For this review, use the dimensioned drawing (mm, ordinates from the lowest corner) and the shaded views. Round coordinates to 2 decimals unless told otherwise and drop trailing zeros. Write each loop counter-clockwise with the first axis right and the second up, starting at its lowest first coordinate (ties: lowest second). Pieces come first, ordered by that corner, then holes. Notation, with made-up numbers: (88.25, 44) - (97.25, 44) arc R7 cw to (97.25, 51) - close; hole circle Ø1 at (53, 46). An arc over 180 degrees is marked (long way). Return JSON: item names as keys, results as strings.
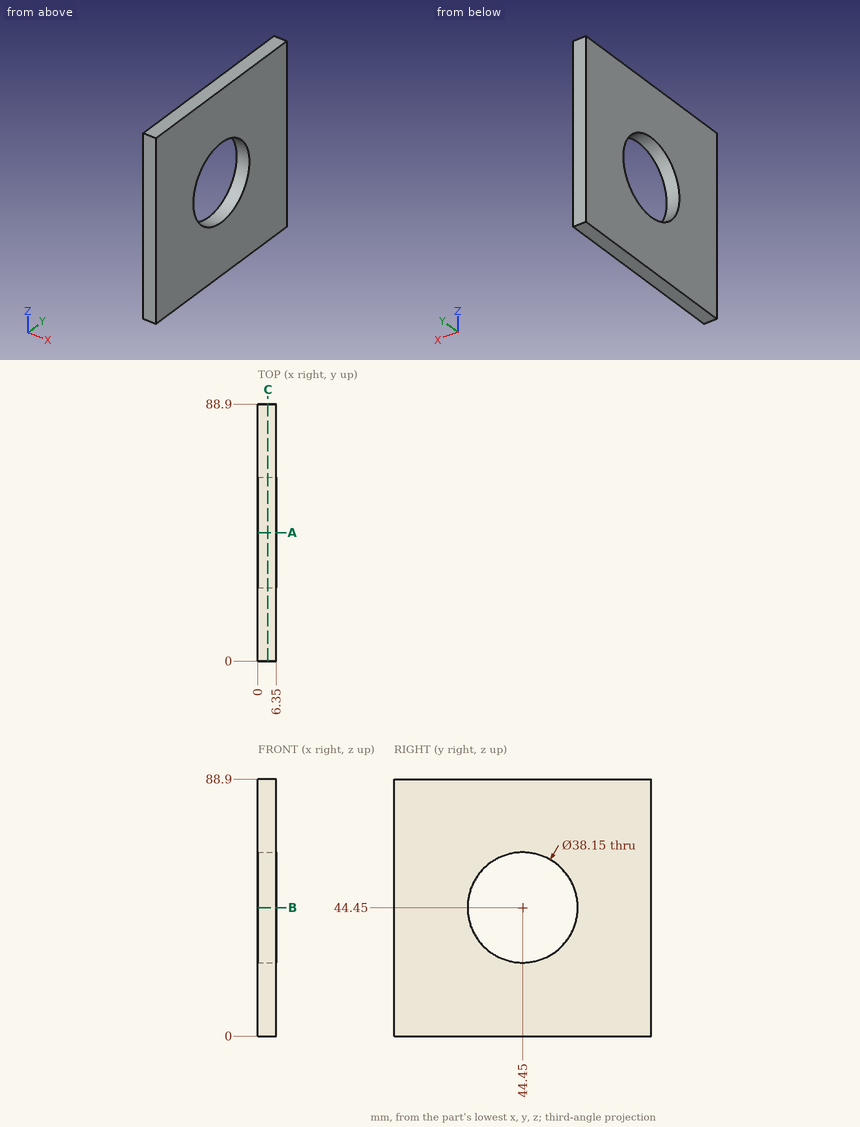
(1) Clearance check with flat-ended pins moving along their axes: pin 1 Ø2 at (x, z) = (2.5, 51) entering from -Y; pin 2 Ø3 at (y, z) = (43, 60) entering from -X. State where each tip first meets the part, or that it passes through.
Filled in:
{"pin 1": "stops at y = 0", "pin 2": "passes through"}
(2) Add section C-C (x = 3.5). Write out the cut boundary in (y, z) (3 decimals).
Filled in:
{"outline": "(0, 0) - (88.9, 0) - (88.9, 88.9) - (0, 88.9) - close; hole circle Ø38.15 at (44.45, 44.45)"}
(3) Wall thickness on line 1 (Z direction, x = 2, y = 44.45) (3 decimals); line 2 (Y direction, x = 2, z = 52); line 3 (Z direction, x = 6.25, y = 38): over which ranges is each line inside the solid? List them lowest first.
Filled in:
{"line 1": "z = 0 to 25.375, 63.525 to 88.9", "line 2": "y = 0 to 26.93, 61.97 to 88.9", "line 3": "z = 0 to 26.5, 62.4 to 88.9"}
(4) Add section A-A (y = 44.45). Write out the cut boundary in (x, z) (3 decimals), plus the area to 3 significant figures.
Filled in:
{"outline": "(0, 0) - (6.35, 0) - (6.35, 25.375) - (0, 25.375) - close; (0, 63.525) - (6.35, 63.525) - (6.35, 88.9) - (0, 88.9) - close", "area": "322 mm2"}
